from build123d import *

# Parameters (mm, degrees)
SKETCH_1_W      = 25
SKETCH_1_H      = 150
EXTRUDE_1_DEPTH = 2.5
CHAMFER_1_SIZE  = 10


with BuildPart() as part:
    # Эскиз1 → Бобышка-Вытянуть1 (new, symmetric)
    with BuildSketch(Plane.XY):
        with Locations((12.5, 75)):
            Rectangle(SKETCH_1_W, SKETCH_1_H)
    extrude(amount=EXTRUDE_1_DEPTH, both=True)

    # Фаска1
    chamfer_1_edges = [part.edges().sort_by_distance(p)[0] for p in [
        (0, 0, 0),
        (0, 150, 0),
    ]]
    chamfer(chamfer_1_edges, length=CHAMFER_1_SIZE)


solid = part.part
Could you check a few things on this model? Use its own coordinates, in mm. Give positions to 0.01 mm unless a question says otherwise; leave off trailing zeros. Loops run counter-clockwise (first coordinate to the right, second up) from the corner with the lowest first, then second, coordinate; pieces in that order, holes last. Notation, with made-up numbers: M 6.25,74.5 L 50.25,74.5 A21 ccw 50.25,108.5 Z; hole C -17,-15 d8. An arc over 180 degrees is marked long. Answer as a JSON object with one key per item and string values.
Q1. Suppose I cut it at C-C, the plane x = 3. List the corners of the cut face in (y, z) for me.
Values found:
{"outline": "M 7,-2.5 L 143,-2.5 L 143,2.5 L 7,2.5 Z"}
Q2. Suppose I cut it at B-B, the plane x = 8.5. List the corners of the cut face in (y, z) for me, plus the area to 3 significant figures.
Values found:
{"outline": "M 1.5,-2.5 L 148.5,-2.5 L 148.5,2.5 L 1.5,2.5 Z", "area": "735 mm²"}
Q3. Suppose I cut it at A-A, the plane z = 1.3. List the corners of the cut face in (x, y) for me.
Values found:
{"outline": "M 0,10 L 10,0 L 25,0 L 25,150 L 10,150 L 0,140 Z"}
Q4. If I drill on probe 1 along X at (y, z) = (7.5, -1.35); probe 2 along Y at (x, z) = (9, 0.1); probe 3 along Y at (x, z) = (4, -0.85), over which ranges is the centre line in solid material (lowest first)? Write a range as [from, to].
Values found:
{"probe 1": "x = [2.5, 25]", "probe 2": "y = [1, 149]", "probe 3": "y = [6, 144]"}
